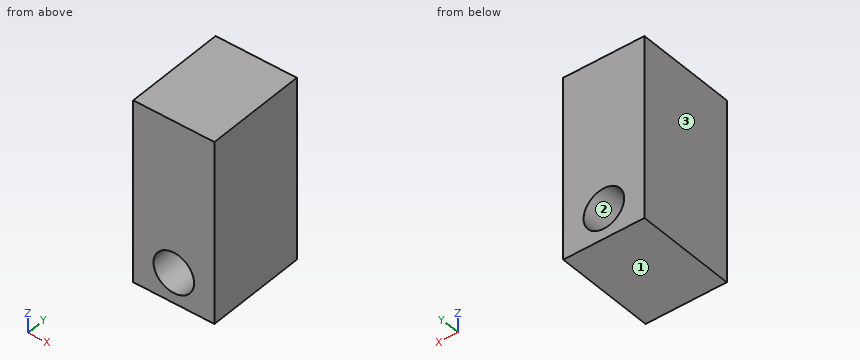
from build123d import *

# Parameters (mm, degrees)
SKETCH1_W           = 40
SKETCH1_H           = 50
BOSS_EXTRUDE1_DEPTH = 90
CUT_EXTRUDE1_REACH  = 106.881
SKETCH2_R           = 10


with BuildPart() as part:
    # Sketch1 → Boss-Extrude1 (new body)
    with BuildSketch(Plane.XY):
        Rectangle(SKETCH1_W, SKETCH1_H)
    extrude(amount=BOSS_EXTRUDE1_DEPTH)

    # Sketch2 → Cut-Extrude1 (cut, up to next)
    with BuildSketch(Plane(origin=(0, 25, 0), x_dir=(1, 0, 0), z_dir=(0, 1, 0)), mode=Mode.PRIVATE) as cut_extrude1_sk1:
        with Locations(Location((0, -15, 0), (0, 0, 180))):
            Circle(SKETCH2_R)
    cut_extrude1_tool1 = extrude(cut_extrude1_sk1.sketch, amount=-CUT_EXTRUDE1_REACH, mode=Mode.PRIVATE) & part.part
    add(cut_extrude1_tool1.solids().sort_by_distance((0, 25, 15))[0], mode=Mode.SUBTRACT)


solid = part.part
Design review of the part built by this model. Coordinates are the model's own, in mm. Face numbers are marked on the shaded views. Round coordinates to 2 decimals unless told otherwise and drop trailing zeros. Write each loop counter-clockwise with the first axis right and the second up, starting at its lowest first coordinate (ties: lowest second). Pieces come first, ordered by that corner, then holes. Notation, with made-up numbers: (26, 40.25) - (73, 40.25) arc R37 ccw to (73, 78.25) - close; hole circle Ø3 at (87, -39). An arc over 180 degrees is marked (long way). Use a Markdown table: item, result. Add a question column.
1. We need section A-A (z = 15). State the section outline as (x, y) points, then the cut area to 3 significant figures.
2. We need section B-B (x = 0). State the section outline as (y, z) points, then the cut area to 3 significant figures.
3. Wall thickness on probe 1 along Z at (x, y) = (0, 1); probe 2 along Z at (x, y) = (2, -5); probe 3 along X at (y, z) = (-8.5, 13.5): over which ranges is each line inside the solid? List them lowest first.
4. We need section C-C (y = 7). State the section outline as (x, z) points.
5. Mouldability with a two-part tool opening along Z and no side actions: class the marked faces 1, 2 and 3 as +Z half, -Z half, draft (parallel to the pull), parting line (faces both ways), or undercut.
Output:
| question | item | result |
|---|---|---|
| 1 | outline | (-20, -25) - (-10, -25) - (-10, 25) - (-20, 25) - close; (10, -25) - (20, -25) - (20, 25) - (10, 25) - close |
| 1 | area | 1,000 mm2 |
| 2 | outline | (-25, 0) - (25, 0) - (25, 5) - (-25, 5) - close; (-25, 25) - (25, 25) - (25, 90) - (-25, 90) - close |
| 2 | area | 3,500 mm2 |
| 3 | probe 1 | z = 0 to 5, 25 to 90 |
| 3 | probe 2 | z = 0 to 5.2, 24.8 to 90 |
| 3 | probe 3 | x = -20 to -9.89, 9.89 to 20 |
| 4 | outline | (-20, 0) - (20, 0) - (20, 90) - (-20, 90) - close; hole circle Ø20 at (0, 15) |
| 5 | face 1 | -Z half |
| 5 | face 2 | undercut |
| 5 | face 3 | draft |
